Build history of the part. All positions in model axes, mm. Round coordinates to 2 decimals unless told otherwise and drop trailing zeros. Loops run counter-clockwise (first coordinate to the right, second up) from the corner with the lowest first, then second, coordinate; pieces in that order, holes last. Notation, with made-up numbers: (-35, 28) - (16, 28) arc R17 ccw to (16, 54) - close; hole circle Ø9 at (38.25, -38.5). An arc over 180 degrees is marked (long way). One line per question, with ' | ' between items. Start each with the question number.
from build123d import *

# Parameters (mm, degrees)
SKETCH1_R           = 10
BOSS_EXTRUDE1_DEPTH = 10
SKETCH3_R           = 15
BOSS_EXTRUDE3_DEPTH = 10
SKETCH4_R           = 5
CUT_EXTRUDE1_DEPTH  = 20


with BuildPart() as part:
    # Sketch1 → Boss-Extrude1 (new body)
    with BuildSketch(Plane(origin=(0, 0, 0), x_dir=(0, 0, -1), z_dir=(1, 0, 0))):
        with BuildLine():
            ThreePointArc((22.040471077, -91.799052281), (0, -55), (-22.040471077, -91.799052281))
            ThreePointArc((-22.040471077, -91.799052281), (-7.5, -153.539335996), (-25.58571686, -214.33567452))
            ThreePointArc((-25.58571686, -214.33567452), (0, -260), (25.58571686, -214.33567452))
            ThreePointArc((25.58571686, -214.33567452), (7.5, -153.539335996), (22.040471077, -91.799052281))
        make_face()
        with Locations((0, -230)):
            Circle(SKETCH1_R, mode=Mode.SUBTRACT)
    extrude(amount=BOSS_EXTRUDE1_DEPTH)

    # Sketch3 → Boss-Extrude3 (add)
    with BuildSketch(Plane.ZY):
        with Locations((0, -80)):
            Circle(SKETCH3_R)
    extrude(amount=BOSS_EXTRUDE3_DEPTH)

    # Sketch4 → Cut-Extrude1 (cut)
    with BuildSketch(Plane.ZY.offset(10)):
        with Locations((0, -80)):
            Circle(SKETCH4_R)
    extrude(amount=-CUT_EXTRUDE1_DEPTH, mode=Mode.SUBTRACT)


solid = part.part
1) Drop flat-ended pins along their axis: pin 1 (8 mm diameter, centred on x = 6, z = -16.5, fed in from +Y); pin 2 (5 mm diameter, centred on x = 7, z = -6.5, fed in from -Y); pin 3 (6 mm diameter, centred on x = -6.5, z = 11, fed in from -Y). Give the stop position or say it passes through.
2) Saw through at C-C on z = -13. Write the cut outline in (x, y), and give its area (3 significant figures).
3) Saw through at A-A on y = -230. Write the cut outline in (x, z), and give its area (3 significant figures).
4) Saw through at B-B on z = 0. Write the cut outline in (x, y).
5) Two-plate mould, pull along Y, no slides. Class faces 1 (the flat face through (-10, -76, -4)), 2 (the cylindrical face through (4.93, -152.642, 7.477)), 3 (the cylindrical face through (-4.93, -94.643, -3.252)): +Y half, -Y half, draft (parallel to the pull), parting line (faces both ways), or undercut.
6) Saw through at D-D on x = 4. Write the cut outline in (y, z), and give its area (3 significant figures).
7) Wall check: line 1 (Y direction, x = -2.25, z = 0); line 2 (X direction, y = -238.5, z = 21); line 3 (Y direction, x = 3.75, z = 19). Give the ranges that are in metal, low to high. Write a range as [from, to].
Answer key:
1) pin 1: y = -58.35 | pin 2: y = -259.73 | pin 3: y = -92.69
2) outline: (-10, -87.48) - (0, -87.48) - (0, -113.4) - (10, -113.4) - (10, -58.65) - (0, -58.65) - (0, -72.52) - (-10, -72.52) - close; (0, -257.04) - (10, -257.04) - (10, -186.55) - (0, -186.55) - close | area: 1,400 mm²
3) outline: (0, -30) - (10, -30) - (10, -10) - (0, -10) - close; (0, 10) - (10, 10) - (10, 30) - (0, 30) - close | area: 400 mm²
4) outline: (-10, -95) - (0, -95) - (0, -220) - (10, -220) - (10, -85) - (-10, -85) - close; (-10, -75) - (10, -75) - (10, -55) - (0, -55) - (0, -65) - (-10, -65) - close; (0, -260) - (10, -260) - (10, -240) - (0, -240) - close
5) face 1: draft | face 2: undercut | face 3: parting line
6) outline: (-214.34, -25.59) arc R123.26 cw to (-91.8, -22.04) arc R25 ccw (long way) to (-91.8, 22.04) arc R123.26 cw to (-214.34, 25.59) arc R30 ccw (long way) to start; hole circle Ø20 at (-230, 0); hole circle Ø10 at (-80, 0) | area: 6,600 mm²
7) line 1: [-95, -85], [-75, -65] | line 2: [0, 10] | line 3: [-253.22, -202.07], [-97.88, -63.75]
